from build123d import *

# Parameters (mm, degrees)
F0_W     = 61.665386
F0_H     = 61.6654
F1_DEPTH = 60
F2_R     = 13.827744
F3_DEPTH = 25
F4_R     = 16.83794
F5_DEPTH = 50
F6_R     = 13.433153
F7_DEPTH = 50


with BuildPart() as f1:
    # F0 (on Top) → F1 (new body)
    with BuildSketch(Plane.XY):
        Rectangle(F0_W, F0_H)
    extrude(amount=F1_DEPTH)

    # F2 (on face) → F3 (cut)
    with BuildSketch(Plane.YZ.offset(30.832693)):
        with Locations((0, 33.078797)):
            Circle(F2_R)
    extrude(amount=-F3_DEPTH, mode=Mode.SUBTRACT)

    # F4 (on face) → F5 (cut)
    with BuildSketch(Plane(origin=(0, 30.8327, 0), x_dir=(-1, 0, 0), z_dir=(0, 1, 0))):
        with Locations((0, 30.424289)):
            Circle(F4_R)
    extrude(amount=F5_DEPTH, mode=Mode.SUBTRACT)

    # F6 (on face) → F7 (cut)
    with BuildSketch(Plane(origin=(0, 30.8327, 0), x_dir=(-1, 0, 0), z_dir=(0, 1, 0))):
        with Locations((0, 30.62848)):
            Circle(F6_R)
    extrude(amount=-F7_DEPTH, mode=Mode.SUBTRACT)


solid = f1.part
Part model, mm, in its own coordinate system. A direction names the side the tool comes from. Coordinates: 2 decimals unless noted, no trailing zeros. Loops run counter-clockwise (first coordinate to the right, second up) from the corner with the lowest first, then second, coordinate; pieces in that order, holes last. Notation, with made-up numbers: M -37.75,8 L 4.25,8 A12 ccw 4.25,15 Z; hole C 57,81.5 d4. An arc over 180 degrees is marked long. Use a Markdown table: item, result. Add a question column.
Q1. Pin check, flat tips, straight feed: P1, Ø13.5, axis at x = 2.5, z = 28.5, coming from the +Y side; P2, Ø1, axis at y = 8, z = 43.5, coming from the +X side; P3, Ø16.5, axis at y = 0, z = 33.08, coming from the +X side. Stop position of each tip, or through.
Q2. Cut at B-B (x = 0). Write the cut outline in (y, z).
Q3. Cut at C-C (y = -4). Write the cut outline in (x, z).
Q4. Mould opens along X. For faces 1 (the flat face through (0, -19.167, 31)), 2 (the flat face through (30.833, 0, 16)), 3 (the flat face through (0, -30.833, 30)) say: +X half, -X half, draft (parallel to the pull), parting line (faces both ways), or undercut.
Q5. Cut at A-A (z = 21). Write the cut outline in (x, y), and give its area (3 significant figures).
Q6. Cut at D-D (x = 16). Write the cut outline in (y, z), and give its area (3 significant figures).
Q7. Which spindle directions (+Z, -Z, +X, -X, +Y, -Y) get a long thin tool onto all of the face, cutting with end or side? Do faces 4 (the flat face through (0, 30.833, 16)), 5 (the cylindrical face through (-12.409, 6.183, 25.484)), 6 (the flat face through (5.833, 0, 44)). Say none if no direction does.
Q8. Probe L1, parallel to Z at x = 17.25, y = 0; L2, parallel to Y at x = 22, z = 32.5; L3, parallel to Z at x = 0, y = 4. List the from-to ranges inside material, lowest first.
Worked out:
| question | item | result |
|---|---|---|
| 1 | P1 | stops at y = -19.17 |
| 1 | P2 | stops at x = 5.83 |
| 1 | P3 | stops at x = -8.12 |
| 2 | outline | M -30.83,0 L 30.83,0 L 30.83,17.2 L -19.17,17.2 L -19.17,44.06 L 30.83,44.06 L 30.83,60 L -30.83,60 Z |
| 3 | outline | M -30.83,0 L 30.83,0 L 30.83,19.84 L 8.01,19.84 A13.43 cw long 5.83,42.73 L 5.83,46.32 L 30.83,46.32 L 30.83,60 L -30.83,60 Z |
| 4 | face 1 | undercut |
| 4 | face 2 | +X half |
| 4 | face 3 | draft |
| 5 | outline | M -30.83,-30.83 L 30.83,-30.83 L 30.83,-6.73 L 9.37,-6.73 L 9.37,-19.17 L -9.37,-19.17 L -9.37,30.83 L -30.83,30.83 Z; M 9.37,6.73 L 30.83,6.73 L 30.83,30.83 L 9.37,30.83 Z |
| 5 | area | 2,580 mm2 |
| 6 | outline | M -30.83,0 L 30.83,0 L 30.83,60 L -30.83,60 Z; hole C 0,33.08 d27.66 |
| 6 | area | 3,100 mm2 |
| 7 | face 4 | +Z, -Z, +X, -X, +Y |
| 7 | face 5 | +Y |
| 7 | face 6 | +X |
| 8 | L1 | z = 0 to 19.25, 46.91 to 60 |
| 8 | L2 | y = -30.83 to -13.82, 13.82 to 30.83 |
| 8 | L3 | z = 0 to 17.2, 44.06 to 60 |
